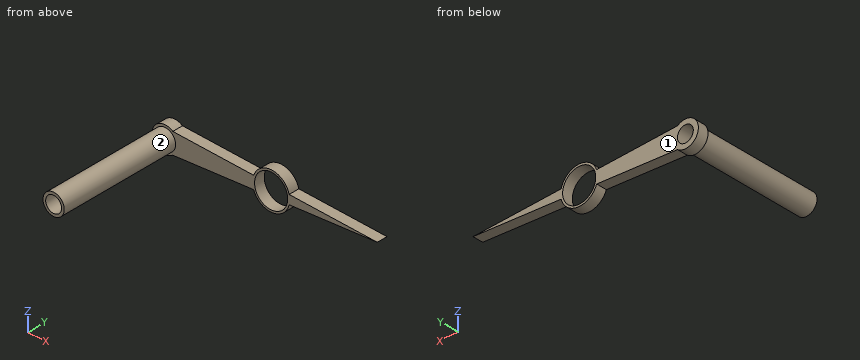
from build123d import *

# Parameters (mm, degrees)
F0_R     = 3.119034
F1_DEPTH = 1
F2_R     = 2
F3_DEPTH = 25
F4_R     = 1.5
F5_DEPTH = 25


with BuildPart() as f1:
    # F0 (on Front) → F1 (new body, symmetric)
    with BuildSketch(Plane.XZ):
        with BuildLine():
            ThreePointArc((1.47637, -1.955206), (2.193126, -1.092106), (2.45, 0))
            ThreePointArc((2.45, 0), (2.193126, 1.092106), (1.47637, 1.955206))
            ThreePointArc((1.47637, 1.955206), (-2.45, 0), (1.47637, -1.955206))
        make_face()
        with BuildLine():
            ThreePointArc((1.47637, 1.955206), (2.193126, 1.092106), (2.45, 0))
            ThreePointArc((2.45, 0), (2.193126, -1.092106), (1.47637, -1.955206))
            Line((1.47637, -1.955206), (16.712802, -1.181905))
            ThreePointArc((16.712802, -1.181905), (16.506782, 0), (16.712802, 1.181905))
            Line((16.712802, 1.181905), (1.47637, 1.955206))
        make_face()
        with BuildLine():
            ThreePointArc((23.38997, 0.843016), (20.177065, 3.488727), (16.712802, 1.181905))
            ThreePointArc((16.712802, 1.181905), (16.506782, 0), (16.712802, -1.181905))
            ThreePointArc((16.712802, -1.181905), (20.177065, -3.488727), (23.38997, -0.843016))
            ThreePointArc((23.38997, -0.843016), (23.46731, -0.424657), (23.493218, 0))
            ThreePointArc((23.493218, 0), (23.46731, 0.424657), (23.38997, 0.843016))
        make_face()
        with Locations((20, 0)):
            Circle(F0_R, mode=Mode.SUBTRACT)
        with BuildLine():
            Line((40, 0), (23.38997, 0.843016))
            ThreePointArc((23.38997, 0.843016), (23.46731, 0.424657), (23.493218, 0))
            ThreePointArc((23.493218, 0), (23.46731, -0.424657), (23.38997, -0.843016))
            Line((23.38997, -0.843016), (40, 0))
        make_face()
    extrude(amount=F1_DEPTH, both=True)

    # F2 (on face) → F3 (join)
    with BuildSketch(Plane(origin=(0, 1, 0), x_dir=(-1, 0, 0), z_dir=(0, 1, 0))):
        Circle(F2_R)
    extrude(amount=-F3_DEPTH)

    # F4 (on face) → F5 (cut)
    with BuildSketch(Plane.XZ.offset(24)):
        Circle(F4_R)
    extrude(amount=-F5_DEPTH, mode=Mode.SUBTRACT)


solid = f1.part
Could you check a few things on this model? Use its own coordinates, in mm. Face numbers are marked on the shaded views. A direction names the side the tool comes from. Coordinates: 2 decimals unless noted, no trailing zeros. Loops run counter-clockwise (first coordinate to the right, second up) from the corner with the lowest first, then second, coordinate; pieces in that order, holes last. Notation, with made-up numbers: (63, -24.5) -> (75, -24.5) arc R24 cw to (75, 11.5) -> close; hole circle Ø4 at (71, 19.5). An arc over 180 degrees is marked (long way). Answer in a Markdown table with one row per item.
(1) Imagine slicing it at B-B (y = -2.5). List the corners of the cut face in (x, z) for me, plus the area to 3 significant figures.
Results found:
| item | result |
|---|---|
| outline | circle Ø4 at (0, 0); hole circle Ø3 at (0, 0) |
| area | 5.50 mm^2 |
(2) For the marked faces 1 and 2, which set-ups out of +Z, -Z, +X, -X, +Y, -Y let a thin tool reach every point of the face, with its end or its side?
Results found:
| item | result |
|---|---|
| face 1 | +Z, -Z, +X, -X, +Y |
| face 2 | -Y |
(3) If I drill on probe 1 along Z at (x, y) = (0, -15.25); probe 2 along Z at (x, y) = (20, -0.2); probe 3 along Y at (x, z) = (11, -0.25), over which ranges is the centre line in solid material (lowest first)?
Results found:
| item | result |
|---|---|
| probe 1 | z = -2 to -1.5, 1.5 to 2 |
| probe 2 | z = -3.49 to -3.12, 3.12 to 3.49 |
| probe 3 | y = -1 to 1 |
(4) Will these pins go through, and if not, where does the flat tip stop? pin 1 Ø2 at (x, z) = (17.5, 2) entering from -Y; pin 2 Ø1 at (y, z) = (-6, 1.5) entering from +X; pin 3 Ø10 at (x, y) = (18.5, -10) entering from +Z.
Results found:
| item | result |
|---|---|
| pin 1 | stops at y = -1 |
| pin 2 | stops at x = 1.73 |
| pin 3 | passes through |
(5) Imagine slicing it at D-D (x = 12.5). List the corners of the cut face in (y, z) for me, plus the area to 3 significant figures.
Results found:
| item | result |
|---|---|
| outline | (-1, -1.4) -> (1, -1.4) -> (1, 1.4) -> (-1, 1.4) -> close |
| area | 5.58 mm^2 |
(6) Imagine slicing it at C-C (x = 0). List the corners of the cut face in (y, z) for me, plus the area to 3 significant figures.
Results found:
| item | result |
|---|---|
| outline | (-24, -2) -> (-1, -2) -> (-1, -2.45) -> (1, -2.45) -> (1, -1.5) -> (-24, -1.5) -> close; (-24, 1.5) -> (1, 1.5) -> (1, 2.45) -> (-1, 2.45) -> (-1, 2) -> (-24, 2) -> close |
| area | 26.8 mm^2 |
(7) Imagine slicing it at A-A (x = 20). List the corners of the cut face in (y, z) for me.
Results found:
| item | result |
|---|---|
| outline | (-1, -3.49) -> (1, -3.49) -> (1, -3.12) -> (-1, -3.12) -> close; (-1, 3.12) -> (1, 3.12) -> (1, 3.49) -> (-1, 3.49) -> close |
